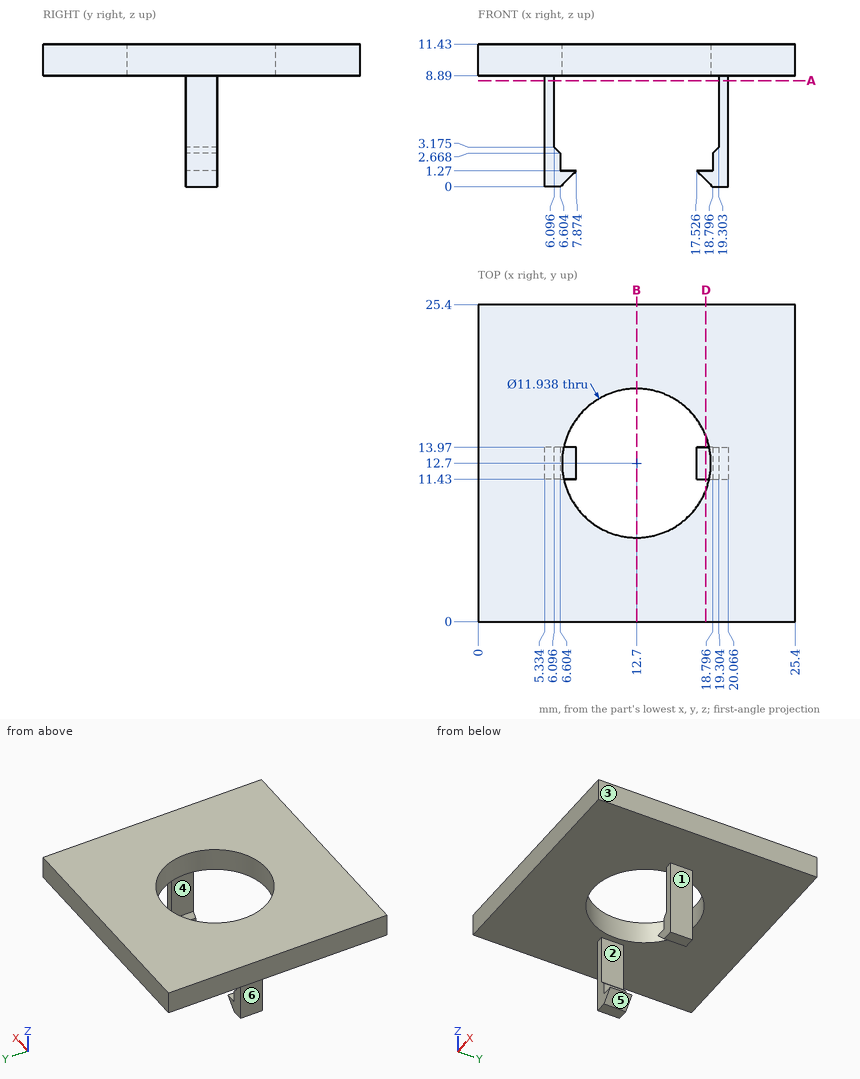
Print and shaded views of the part. All mm, measured from the part's lowest x, y and z. A direction names the side the tool comes from. Round coordinates to 2 decimals unless told otherwise and drop trailing zeros. Write each loop counter-clockwise with the first axis right and the second up, starting at its lowest first coordinate (ties: lowest second). Pieces come first, ordered by that corner, then holes. Notation, with made-up numbers: (72.25, 78) - (99.25, 78) arc R9 cw to (99.25, 91) - close; hole circle Ø3 at (-8.75, 58). An arc over 180 degrees is marked (long way). One line per question, with ' | ' between items.
1. Tool access for the marked faces 1, 2 and 3: list every direction of +Z, -Z, +X, -X, +Y, -Y with a clear straight run to the whole face (end or side of a thin tool).
Results are:
face 1: -Z, +X, +Y, -Y | face 2: +Y, -Y | face 3: +Z, -Z, +X, +Y, -Y
2. Band-saw the part on B-B, the plane x = 12.7. Write the cut outline in (y, z).
Results are:
outline: (0, 8.89) - (6.73, 8.89) - (6.73, 11.43) - (0, 11.43) - close; (18.67, 8.89) - (25.4, 8.89) - (25.4, 11.43) - (18.67, 11.43) - close
3. Mould opens along Z. For the marked faces 4, 5 and 6 say: released by +Z, released by -Z, zero draft, split by the parting line, or undercut.
Results are:
face 4: undercut | face 5: released by -Z | face 6: zero draft
4. Band-saw the part on D-D, the plane x = 18.25. Write the cut outline in (y, z) (1 decimal).
Results are:
outline: (0, 8.9) - (10.5, 8.9) - (10.5, 11.4) - (0, 11.4) - close; (11.4, 0.5) - (14, 0.5) - (14, 1.3) - (11.4, 1.3) - close; (14.9, 8.9) - (25.4, 8.9) - (25.4, 11.4) - (14.9, 11.4) - close
5. Band-saw the part on A-A, the plane z = 8.5. Write the cut outline in (x, y) (1 decimal).
Results are:
outline: (5.3, 11.4) - (6.1, 11.4) - (6.1, 14) - (5.3, 14) - close; (19.3, 11.4) - (20.1, 11.4) - (20.1, 14) - (19.3, 14) - close
6. Drop flat-ended pins along their axis: pin 1 Ø6 at (y, z) = (7, 5) entering from +X; pin 2 Ø3 at (y, z) = (12, 6.5) entering from +X; pin 3 Ø2 at (x, y) = (16.5, 17.5) entering from -Z; pin 4 Ø0.6 at (x, y) = (18, 12.5) entering from +Z. Give the stop position or say it passes through.
Results are:
pin 1: through | pin 2: x = 20.07 | pin 3: z = 8.89 | pin 4: z = 1.27
7. Drill centre lines: line 1 along Y through (x, z) = (12.7, 10.6); line 2 along Z through (x, y) = (13, 21.5); line 3 along X through (y, z) = (13.75, 7) (1 decimal). Where is each one in solid material? Low to high. Write a range as from..to.
Results are:
line 1: 0..6.73, 18.67..25.4 | line 2: 8.89..11.43 | line 3: 5.3..6.1, 19.3..20.1
